Could you check a few things on this model? Use its own coordinates, in mm. A direction names the side the tool comes from. Give positions to 0.01 mm unless a question says otherwise; leave off trailing zeros. Write each loop counter-clockwise with the first axis right and the second up, starting at its lowest first coordinate (ties: lowest second). Pieces come first, ordered by that corner, then holes. Notation, with made-up numbers: (64.5, -16.5) - (100.5, -16.5) arc R17 cw to (100.5, 16.5) - close; hole circle Ø3 at (16, 46). An arc over 180 degrees is marked (long way). Answer in a Markdown table with one row per item.
from build123d import *

# Parameters (mm, degrees)
F0_W     = 20
F0_H     = 20
F1_DEPTH = 20
F2_W     = 16
F2_H     = 16
F3_DEPTH = 15
F4_W     = 16
F4_H     = 16
F5_DEPTH = 15
F6_W     = 16
F6_H     = 16
F7_DEPTH = 15


with BuildPart() as f1:
    # F0 (on Front) → F1 (new body)
    with BuildSketch(Plane.XZ):
        with Locations((10, -10)):
            Rectangle(F0_W, F0_H)
    extrude(amount=F1_DEPTH)

    # F2 (on face) → F3 (join)
    with BuildSketch(Plane.XZ.offset(20)):
        with Locations((10, -10)):
            Rectangle(F2_W, F2_H)
    extrude(amount=F3_DEPTH)

    # F4 (on face) → F5 (join)
    with BuildSketch(Plane.YZ.offset(20)):
        with Locations((-10, -10)):
            Rectangle(F4_W, F4_H)
    extrude(amount=F5_DEPTH)

    # F6 (on face) → F7 (join)
    with BuildSketch(Plane.XY):
        with Locations((10, -10)):
            Rectangle(F6_W, F6_H)
    extrude(amount=F7_DEPTH)


solid = f1.part
1) If I drill on line 1 (Z direction, x = 29.5, y = -16); line 2 (X direction, y = -19, z = -15), over which ranges is the centre line in solid material (lowest first)?
Check values:
| item | result |
|---|---|
| line 1 | z = -18 to -2 |
| line 2 | x = 0 to 20 |
2) On a 3-axis mill with a long thin cutter (end or side, diameter ignored), from which of +Z, -Z, +X, -X, +Y, -Y can I reach the whole of each face in a straight line? I mean faces 4 (the face through (10, -2, 7)), 5 (the face through (27, -10, -2)), 6 (the face through (27, -10, -18)). Say none if no direction works.
Check values:
| item | result |
|---|---|
| face 4 | +Z, +X, -X, +Y |
| face 5 | +Z, +X, +Y, -Y |
| face 6 | -Z, +X, +Y, -Y |
3) Will these pins go through, and if not, where does the flat tip stop? P1, Ø7.5, axis at x = 28, z = -10, coming from the +Y side; P2, Ø1.5, axis at x = 25, y = -5, coming from the -Z side; P3, Ø5, axis at x = 20.5, y = -15, coming from the -Z side; P4, Ø16.5, axis at x = 12, z = 6.5, coming from the -Y side.
Check values:
| item | result |
|---|---|
| P1 | stops at y = -2 |
| P2 | stops at z = -18 |
| P3 | stops at z = -20 |
| P4 | stops at y = -20 |
4) Imagine slicing it at B-B (z = -6). List the corners of the cut face in (x, y) for me.
Check values:
| item | result |
|---|---|
| outline | (0, -20) - (2, -20) - (2, -35) - (18, -35) - (18, -20) - (20, -20) - (20, -18) - (35, -18) - (35, -2) - (20, -2) - (20, 0) - (0, 0) - close |
5) Imagine slicing it at A-A (y = -6.5). List the corners of the cut face in (x, z) for me, then the cut area to 3 significant figures.
Check values:
| item | result |
|---|---|
| outline | (0, -20) - (20, -20) - (20, -18) - (35, -18) - (35, -2) - (20, -2) - (20, 0) - (18, 0) - (18, 15) - (2, 15) - (2, 0) - (0, 0) - close |
| area | 880 mm2 |
6) We'd pull the mould along X, two halves only. Please class faces 1 (the face through (35, -10, -10)), 2 (the face through (27, -2, -10)), 3 (the face through (0, -10, -10)): +X half, -X half, draft (parallel to the pull), parting line (faces both ways), or undercut.
Check values:
| item | result |
|---|---|
| face 1 | +X half |
| face 2 | draft |
| face 3 | -X half |
7) Imagine slicing it at D-D (y = -19). List the corners of the cut face in (x, z) for me.
Check values:
| item | result |
|---|---|
| outline | (0, -20) - (20, -20) - (20, 0) - (0, 0) - close |
8) Imagine slicing it at C-C (x = 31). List the corners of the cut face in (y, z) for me.
Check values:
| item | result |
|---|---|
| outline | (-18, -18) - (-2, -18) - (-2, -2) - (-18, -2) - close |
